For this review, use the dimensioned drawing (mm, ordinates from the lowest corner) and the shaded views. Round coordinates to 2 decimals unless told otherwise and drop trailing zeros. Write each loop counter-clockwise with the first axis right and the second up, starting at its lowest first coordinate (ties: lowest second). Pieces come first, ordered by that corner, then holes. Notation, with made-up numbers: (81.25, 25.5) -> (108.25, 25.5) arc R14 ccw to (108.25, 34.5) -> close; hole circle Ø5 at (82, 48). An arc over 180 degrees is marked (long way). Answer in a Markdown table with one row per item. Add a question column.
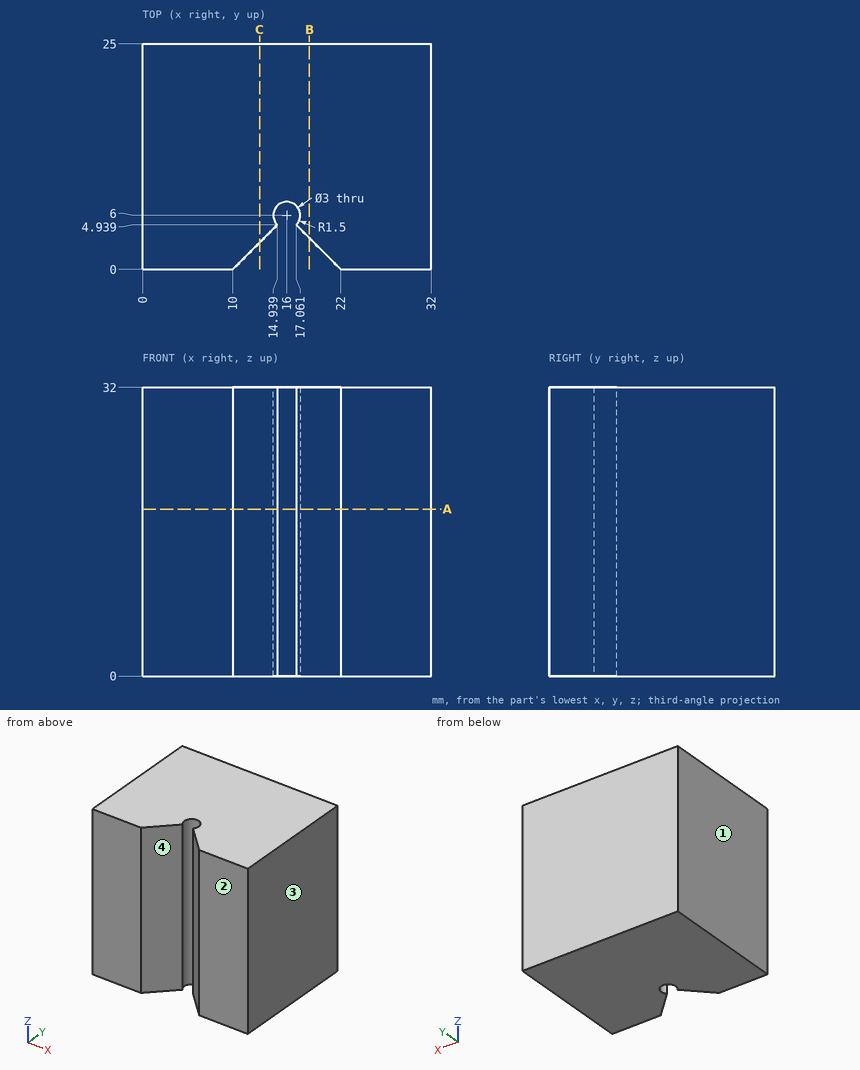
1. The part is to be moulded in two halves that separate along X. For the marked faces 1, 2, 3 and 4, say which applies: pulls with the +X half, pulls with the -X half, needs draft (parallel to the pull), parting line crosses it, or undercut.
2. Clearance check with a flat-ended pin moving along its axis: pin 1 Ø2.5 at (x, y) = (16, 6) entering from +Z. State where the tip first meets the part, or that it passes through.
3. We need section C-C (x = 13). Write out the cut boundary in (y, z).
4. For L1, parallel to X at y = 6, z = 15.5; L2, parallel to Y at x = 16, z = 19; L3, parallel to X at y = 2.25, z = 28, list the stretches that pass through material, from the lowest coordinate up. Write a range as [from, to].
5. We need section A-A (z = 18.5). Write out the cut boundary in (x, y).
6. We need section B-B (x = 18.5). Write out the cut boundary in (y, z).
Response:
| question | item | result |
|---|---|---|
| 1 | face 1 | pulls with the -X half |
| 1 | face 2 | needs draft |
| 1 | face 3 | pulls with the +X half |
| 1 | face 4 | undercut |
| 2 | pin 1 | through |
| 3 | outline | (3, 0) -> (25, 0) -> (25, 32) -> (3, 32) -> close |
| 4 | L1 | [0, 14.5], [17.5, 32] |
| 4 | L2 | [7.5, 25] |
| 4 | L3 | [0, 12.25], [19.75, 32] |
| 5 | outline | (0, 0) -> (10, 0) -> (14.94, 4.94) arc R1.5 cw (long way) to (17.06, 4.94) -> (22, 0) -> (32, 0) -> (32, 25) -> (0, 25) -> close |
| 6 | outline | (3.5, 0) -> (25, 0) -> (25, 32) -> (3.5, 32) -> close |
